The listing builds one solid part. Answer for the finished solid, in the listing's coordinates (mm). Face numbers are marked on the shaded views. A direction names the side the tool comes from. Give positions to 0.01 mm unless a question says otherwise; leave off trailing zeros. Order: outer loops, then holes, each group sorted by start corner. A loop starts at its lowest first (then second) coordinate and runs counter-clockwise, first axis right, second up. Notation, with made-up numbers: (62.5, -28.75) -> (67.5, -28.75) arc R10 ccw to (67.5, -21.75) -> close; hole circle Ø7 at (31.25, -22). An arc over 180 degrees is marked (long way). Answer as a JSON object with one key per item and string values. Group by question number.
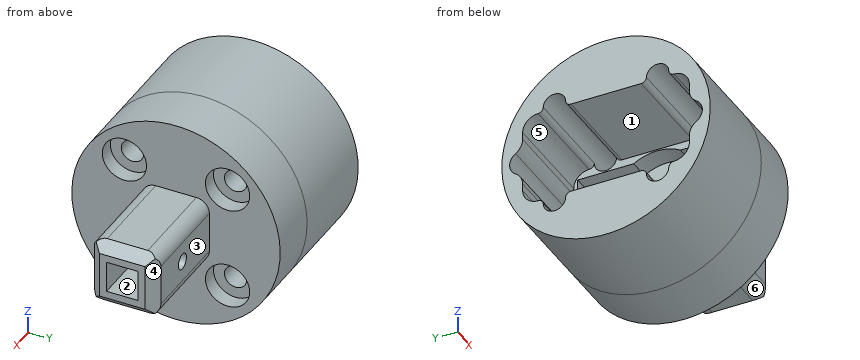
```python
from build123d import *

# Parameters (mm, degrees)
SKETCH_1_R               = 20
EXTRUDE_1_DEPTH          = 10
SKETCH_2_W               = 15
SKETCH_2_H               = 30.5
CUT_EXTRUDE_1_DEPTH      = 4
SKETCH_3_R               = 8.75
CUT_EXTRUDE_2_DEPTH      = 4
EXTRUDE_START            = 19
SKETCH_4_R               = 20
SKETCH_4_W               = 18
SKETCH_4_H               = 32
EXTRUDE_2_DEPTH          = 19
FILLET_1_R               = 3
SKETCH_5_R               = 2.5
CUT_EXTRUDE_3_DEPTH      = 20
FILLET_2_R               = 3
SKETCH_6_R               = 2.15
CUT_EXTRUDE_4_DEPTH      = 43
FILLET_3_R               = 1
SKETCH_7_R               = 4.25
CUT_EXTRUDE_5_DEPTH      = 3
PATTERN_CIRCULAR_1_COUNT = 4
SKETCH_8_W               = 12.8
SKETCH_8_H               = 12.8
EXTRUDE_3_DEPTH          = 20
SKETCH_9_W               = 6
SKETCH_9_H               = 6
CUT_EXTRUDE_6_DEPTH      = 35
SKETCH_10_W              = 3
SKETCH_10_H              = 15
CUT_EXTRUDE_7_DEPTH      = 5
SKETCH_11_R              = 2.5
CUT_EXTRUDE_8_DEPTH      = 5
SKETCH_12_R              = 1.5
CUT_EXTRUDE_9_DEPTH      = 17
CHAMFER_1_SIZE           = 2
FILLET_4_R               = 3
FILLET_5_R               = 2.5


with BuildPart() as part:
    # 草图1 → 凸台-拉伸1 (new body)
    with BuildSketch(Plane(origin=(0, 0, 0), x_dir=(0, 0, -1), z_dir=(1, 0, 0))):
        Circle(SKETCH_1_R)
    extrude(amount=EXTRUDE_1_DEPTH)

    # 草图2 → 切除-拉伸1 (cut)
    with BuildSketch(Plane.ZY):
        Rectangle(SKETCH_2_W, SKETCH_2_H)
    extrude(amount=-CUT_EXTRUDE_1_DEPTH, mode=Mode.SUBTRACT)

    # 草图3 → 切除-拉伸2 (cut)
    with BuildSketch(Plane.ZY.offset(-4)):
        Circle(SKETCH_3_R)
    extrude(amount=CUT_EXTRUDE_2_DEPTH, mode=Mode.SUBTRACT)

    # 草图4 → 凸台-拉伸2 (add)
    with BuildSketch(Plane.ZY.offset(EXTRUDE_START)):
        Circle(SKETCH_4_R)
        Rectangle(SKETCH_4_W, SKETCH_4_H, mode=Mode.SUBTRACT)
    extrude(amount=-EXTRUDE_2_DEPTH)

    # 圆角1
    fillet_1_edges = [part.edges().sort_by_distance(p)[0] for p in [
        (-9.5, 16, 9),
        (-9.5, 16, -9),
        (-9.5, -16, -9),
        (-9.5, -16, 9),
    ]]
    fillet(fillet_1_edges, radius=FILLET_1_R)

    # 草图5 → 切除-拉伸3 (cut)
    with BuildSketch(Plane.ZY.offset(19)):
        with Locations((0, -16)):
            Circle(SKETCH_5_R)
        with Locations((0, 16)):
            Circle(SKETCH_5_R)
    extrude(amount=-CUT_EXTRUDE_3_DEPTH, mode=Mode.SUBTRACT)

    # 圆角2
    # the kernel refuses this fillet: 3 mm, written as the material it takes off along each edge
    with BuildSketch(Plane(origin=(-24.274430572, -16, 2.5), x_dir=(0, -0.9586814917396833, -0.2844816292764363), z_dir=(1, 0, 0))) as fillet_2_piece_1:
        with BuildLine():
            CenterArc((2.275853034, -2.876044475), FILLET_2_R, 106.527865575, 56.944268849)
            Line((-0.600191441, -2.022599587), (0, 0))
            ThreePointArc((0, 0), (0.711204073, -0.103296271), (1.422408146, 0))
        make_face()
    extrude(amount=24.274430572, mode=Mode.SUBTRACT)
    with BuildSketch(Plane(origin=(0, -16, -2.5), x_dir=(0, 0, -1), z_dir=(-1, 0, 0))) as fillet_2_piece_2:
        with BuildLine():
            CenterArc((2.109772229, 3), FILLET_2_R, 213.055731151, 56.944268849)
            ThreePointArc((-0.404648987, 1.363636364), (-0.103296271, 0.711204073), (0, 0))
            Line((0, 0), (2.109772229, 0))
        make_face()
    extrude(amount=24.274430572, mode=Mode.SUBTRACT)
    with BuildSketch(Plane(origin=(0, 16, -2.5), x_dir=(0, 0.9586814917396834, 0.2844816292764354), z_dir=(-1, 0, 0))) as fillet_2_piece_3:
        with BuildLine():
            CenterArc((2.275853034, 2.876044475), FILLET_2_R, 196.527865575, 56.944268849)
            Line((-0.600191441, 2.022599587), (0, 0))
            ThreePointArc((0, 0), (0.711204073, 0.103296271), (1.422408146, 0))
        make_face()
    extrude(amount=24.274430572, mode=Mode.SUBTRACT)
    with BuildSketch(Plane(origin=(-24.274430572, 16, 2.5), x_dir=(0, 0, 1), z_dir=(1, 0, 0))) as fillet_2_piece_4:
        with BuildLine():
            CenterArc((2.109772229, -3), FILLET_2_R, 90, 56.944268849)
            ThreePointArc((-0.404648987, -1.363636364), (-0.103296271, -0.711204073), (0, 0))
            Line((0, 0), (2.109772229, 0))
        make_face()
    extrude(amount=24.274430572, mode=Mode.SUBTRACT)

    # 草图6 → 切除-拉伸4 (cut)
    with BuildSketch(Plane(origin=(10, 0, 0), x_dir=(0, 0, -1), z_dir=(1, 0, 0))):
        with Locations((9.899494937, -9.899494937)):
            Circle(SKETCH_6_R)
        with Locations((-9.899494937, -9.899494937)):
            Circle(SKETCH_6_R)
        with Locations((-9.899494937, 9.899494937)):
            Circle(SKETCH_6_R)
        with Locations((9.899494937, 9.899494937)):
            Circle(SKETCH_6_R)
    extrude(amount=-CUT_EXTRUDE_4_DEPTH, mode=Mode.SUBTRACT)

    # 圆角3
    # the kernel refuses this fillet: 1 mm, written as the material it takes off along each edge
    with BuildSketch(Plane(origin=(-21.98900269, -7.946699797, 9), x_dir=(0, 0.1985408891964352, 0.9800926054802622), z_dir=(1, 0, 0)), Plane(origin=(-21.98900269, 7.946699797, -9), x_dir=(0, -0.19854088919647347, -0.9800926054802545), z_dir=(1, 0, 0))) as fillet_3_piece_1:
        with BuildLine():
            CenterArc((1.217468306, -0.973258884), FILLET_3_R, 103.280057781, 88.171589383)
            Line((0.237375701, -1.171799774), (0, 0))
            ThreePointArc((0, 0), (0.493878653, -0.057493399), (0.987757305, 0))
        make_face()
    extrude(amount=21.98900269, mode=Mode.SUBTRACT)
    with BuildSketch(Plane(origin=(-21.959087911, -11.852290077, 9), x_dir=(0, -0.999999983485678, -0.00018173784322620402), z_dir=(1, 0, 0)), Plane(origin=(-21.959087911, 11.852290077, -9), x_dir=(0, 0.9999999834856781, 0.00018173784322619477), z_dir=(1, 0, 0))) as fillet_3_piece_2:
        with BuildLine():
            CenterArc((1.195428513, -0.999930456), FILLET_3_R, 90.675724778, 87.490671362)
            Line((0.195940547, -0.967933494), (0.09599175, -0.964733798))
            ThreePointArc((0.09599175, -0.964733798), (0.056286672, -0.492404834), (-0.090835283, -0.041820466))
            Line((-0.090835283, -0.041820466), (1.8174e-05, 0.099999998))
            ThreePointArc((1.8174e-05, 0.099999998), (1.147728078, 0.099791416), (1.182455829, 0.099993046))
            Line((1.182455829, 0.099993046), (1.183635164, 0))
        make_face()
    extrude(amount=21.959087911, mode=Mode.SUBTRACT)
    with BuildSketch(Plane(origin=(-21.959087911, -11.852290077, -9), x_dir=(0, -0.19858553154825268, -0.98008356105982), z_dir=(1, 0, 0)), Plane(origin=(-21.959087911, 11.852290077, 9), x_dir=(0, 0.19858553154822475, 0.9800835610598256), z_dir=(1, 0, 0))) as fillet_3_piece_3:
        with BuildLine():
            CenterArc((1.217233349, -0.973269347), FILLET_3_R, 103.277447997, 87.490671362)
            Line((0.234841987, -1.160104066), (0.136602851, -1.178787538))
            ThreePointArc((0.136602851, -1.178787538), (0.129910229, -1.144710182), (-0.098008356, -0.019858553))
            Line((-0.098008356, -0.019858553), (0.022966667, 0.097326935))
            ThreePointArc((0.022966667, 0.097326935), (0.49378334, 0.042529095), (0.964600013, 0.097326935))
            Line((0.964600013, 0.097326935), (0.987566679, 0))
        make_face()
    extrude(amount=21.959087911, mode=Mode.SUBTRACT)
    with BuildSketch(Plane(origin=(-21.98900269, -7.946699797, -9), x_dir=(0, 1, 0), z_dir=(1, 0, 0)), Plane(origin=(-21.98900269, 7.946699797, 9), x_dir=(0, -1, 0), z_dir=(1, 0, 0))) as fillet_3_piece_4:
        with BuildLine():
            CenterArc((1.195601076, -1), FILLET_3_R, 90, 88.171589383)
            ThreePointArc((0.196110214, -0.968093631), (0.154403962, -0.472632025), (0, 0))
            Line((0, 0), (1.195601076, 0))
        make_face()
    extrude(amount=21.98900269, mode=Mode.SUBTRACT)

    # 草图7 → 切除-拉伸5 (cut)
    with BuildSketch(Plane(origin=(10, 0, 0), x_dir=(0, 0, -1), z_dir=(1, 0, 0))):
        with Locations((9.899494937, -9.899494937)):
            Circle(SKETCH_7_R)
    cut_extrude_5 = extrude(amount=-CUT_EXTRUDE_5_DEPTH, mode=Mode.SUBTRACT)

    # 阵列(圆周)1: 切除-拉伸5 ×4 about axis
    pattern_circular_1_axis = Axis((0, 0, 0), (1, 0, 0))
    for i in range(1, PATTERN_CIRCULAR_1_COUNT):
        add(cut_extrude_5.rotate(pattern_circular_1_axis, i * 360 / PATTERN_CIRCULAR_1_COUNT), mode=Mode.SUBTRACT)

    # 草图8 → 凸台-拉伸3 (add)
    with BuildSketch(Plane(origin=(10, 0, 0), x_dir=(0, 0, -1), z_dir=(1, 0, 0))):
        Rectangle(SKETCH_8_W, SKETCH_8_H)
    extrude(amount=EXTRUDE_3_DEPTH)

    # 草图9 → 切除-拉伸6 (cut)
    with BuildSketch(Plane(origin=(30, 0, 0), x_dir=(0, 0, -1), z_dir=(1, 0, 0))):
        Rectangle(SKETCH_9_W, SKETCH_9_H)
    extrude(amount=-CUT_EXTRUDE_6_DEPTH, mode=Mode.SUBTRACT)

    # 草图10 → 切除-拉伸7 (cut)
    with BuildSketch(Plane.ZY.offset(-1)):
        with Locations((0, 10.5)):
            Rectangle(SKETCH_10_W, SKETCH_10_H)
    extrude(amount=-CUT_EXTRUDE_7_DEPTH, mode=Mode.SUBTRACT)

    # 草图11 → 切除-拉伸8 (cut)
    with BuildSketch(Plane.ZY.offset(-1)):
        with Locations((0, 16)):
            Circle(SKETCH_11_R)
    extrude(amount=-CUT_EXTRUDE_8_DEPTH, mode=Mode.SUBTRACT)

    # 草图12 → 切除-拉伸9 (cut)
    with BuildSketch(Plane.XZ.offset(6.4)):
        with Locations(Location((20, 0.05, 0), (0, 0, 270))):
            Circle(SKETCH_12_R)
    extrude(amount=-CUT_EXTRUDE_9_DEPTH, mode=Mode.SUBTRACT)

    # 倒角1
    chamfer_1_edges = [part.edges().sort_by_distance(p)[0] for p in [
        (30, 0, 6.4),
        (30, -6.4, 0),
        (30, 0, -6.4),
        (30, 6.4, 0),
    ]]
    chamfer(chamfer_1_edges, length=CHAMFER_1_SIZE)

    # 圆角4
    fillet_4_edges = [part.edges().sort_by_distance(p)[0] for p in [
        (6, 3, 0),
    ]]
    fillet(fillet_4_edges, radius=FILLET_4_R)

    # 圆角5
    fillet_5_edges = [part.edges().sort_by_distance(p)[0] for p in [
        (19, -6.4, 6.4),
        (19, 6.4, 6.4),
        (19, 6.4, -6.4),
        (19, -6.4, -6.4),
    ]]
    fillet(fillet_5_edges, radius=FILLET_5_R)


solid = part.part
```
(1) A cutting plane is placed at A-A (x = 20). Determine the outline of the cut face in (y, z), and give its area (3 significant figures).
(2) Find the intervals of material crossed by line 1 along Y through (x, z) = (27, -1); line 2 along Y through (x, z) = (8, -7.5); line 3 along Z through (x, y) = (-15.5, 9), in increasing order. Write a range as [from, to].
(3) Flat-ended cylindrical pins translate along their axes: pin 1 Ø6 at (x, y) = (22, -1.5) entering from -Z; pin 2 Ø4.5 at (y, z) = (-16, 0) entering from +X; pin 3 Ø1 at (x, z) = (-11, -11) entering from -Y. Find the tip coordinate at first contact, or state that the pin passes through.
(4) A cutting plane is placed at B-B (y = 2). Determine the outline of the cut face in (x, z), and give its area (3 significant figures).
(5) For a pull along Y with two mould halves and no side action, classify the marked faces 4, 5 and 6 as +Y half, -Y half, draft (parallel to the pull), parting line (faces both ways), or undercut.
(6) A cutting plane is placed at D-D (y = 11). Determine the outline of the cut face in (x, z), and give its area (3 significant figures).
(7) A cutting plane is placed at C-C (z = 0.05). State how many separate pieces and enclosed holes the cut face has, and give its area (3 significant figures).
(8) Which of the six approach directions +Z, -Z, +X, -X, +Y, -Y give full straight-line access (tool end or side, diameter ignored) to the marked faces 1, 2 and 3?
Check sheet entries:
{
 "1": {"outline": "(-6.4, -3.9) arc R2.5 ccw to (-3.9, -6.4) -> (3.9, -6.4) arc R2.5 ccw to (6.4, -3.9) -> (6.4, -1.45) -> (3, -1.45) -> (3, -3) -> (-3, -3) -> (-3, -1.45) -> (-6.4, -1.45) -> close; (-6.4, 1.55) -> (-3, 1.55) -> (-3, 3) -> (3, 3) -> (3, 1.55) -> (6.4, 1.55) -> (6.4, 3.9) arc R2.5 ccw to (3.9, 6.4) -> (-3.9, 6.4) arc R2.5 ccw to (-6.4, 3.9) -> close", "area": "102 mm2"},
 "2": {"line 1": "y = [-6.4, -3], [3, 6.4]", "line 2": "y = [-18.54, -13.41], [-6.39, 6.39], [13.41, 18.54]", "line 3": "z = [-17.86, -11.85], [11.85, 17.86]"},
 "3": {"pin 1": "stops at z = -6.4", "pin 2": "stops at x = 10", "pin 3": "stops at y = -17.02"},
 "4": {"outline": "(-19, -19.9) -> (10, -19.9) -> (10, -6.4) -> (28, -6.4) -> (30, -4.4) -> (30, -3) -> (4, -3) -> (4, -8.52) -> (0, -8.52) -> (0, -9) -> (-19, -9) -> close; (-19, 9) -> (0, 9) -> (0, 8.52) -> (4, 8.52) -> (4, 3) -> (30, 3) -> (30, 4.4) -> (28, 6.4) -> (10, 6.4) -> (10, 19.9) -> (-19, 19.9) -> close", "area": "840 mm2"},
 "5": {"face 4": "+Y half", "face 5": "undercut", "face 6": "-Y half"},
 "6": {"outline": "(-19, -16.7) -> (10, -16.7) -> (10, -14) -> (7, -14) -> (7, -11.75) -> (-19, -11.75) -> close; (-19, 11.75) -> (7, 11.75) -> (7, 14) -> (10, 14) -> (10, 16.7) -> (-19, 16.7) -> close; (0, -8.05) -> (7, -8.05) -> (7, -5.79) -> (10, -5.79) -> (10, 5.79) -> (7, 5.79) -> (7, 8.05) -> (0, 8.05) -> (0, 7.5) -> (4, 7.5) -> (4, 1.5) -> (6, 1.5) -> (6, -1.5) -> (4, -1.5) -> (4, -7.5) -> (0, -7.5) -> close", "area": "355 mm2"},
 "7": {"separate pieces": "4", "enclosed holes": "0", "area": "361 mm2"},
 "8": {"face 1": "-X", "face 2": "+X, -X", "face 3": "+Z, -Z, +X, +Y"}
}
